Autodesk Inventor part; units mm, degrees
ref_plane "Work Plane2" through (0, 0, 6.858) normal (0, 0, 1) x (1, 0, 0)
ref_plane "YZ Plane" through (0, 0, 0) normal (1, 0, 0) x (0, 1, 0)
ref_plane "XZ Plane" through (0, 0, 0) normal (0, 1, 0) x (-1, 0, 0)
sketch "Sketch1" plane through (0, 0, 0) normal (0, 0, 1) x (1, 0, 0)
  circle A0 centre (0, 0) radius 2.159
  dimension "d0" = 4.318
extrude "Extrusion1" add sketch "Sketch1" along normal blind 15.748
sketch "Sketch2" plane through (0, 0, 15.748) normal (0, 0, 1) x (1, 0, 0)
  circle A0 centre (0, 0) radius 1.275
  dimension "d23" = 2.55
extrude "Extrusion2" cut sketch "Sketch2" against normal blind 15.24
sketch "Sketch6" plane through (0, 0, 15.748) normal (0, 0, 1) x (1, 0, 0)
  line L0 (-1.6256, 0.5334) -> (1.6256, 0.5334)
  line L1 (1.6256, 0.5334) -> (1.6256, -0.5334)
  line L2 (1.6256, -0.5334) -> (-1.6256, -0.5334)
  line L3 (-1.6256, -0.5334) -> (-1.6256, 0.5334)
  point P0 (0, 0)
  dimension "d24" = 0.5334
  dimension "d25" = 0.5334
  dimension "d26" = 1.6256
  dimension "d27" = 1.6256
extrude "Extrusion6" cut sketch "Sketch6" against normal blind 8.89
ref_plane "Work Plane2" through (0, 0, 6.858) normal (0, 0, 1) x (1, 0, 0)
sketch "Sketch7" plane through (0, 0, 6.858) normal (0, 0, 1) x (1, 0, 0)
  line L0 (1.6428, -0.5334) -> (1.1581, -0.5334)
  line L1 (-1.6428, 0.5334) -> (-0.5334, 0.5334)
  arc A0 (1.6428, -0.5334) -> (-0.5334, 1.6428) centre (0, 0) ccw
  arc A1 (-1.6428, 0.5334) -> (0.5334, -1.6428) centre (0, 0) ccw
  line L2 (1.6256, -0.5334) -> (0.5334, -0.5334)
  line L3 (0.5334, -0.5334) -> (0.5334, -1.6428)
  line L4 (-0.5334, 0.5334) -> (-0.5334, 1.6428)
extrude "Extrusion7" cut sketch "Sketch7" along normal blind 5.588
sketch "Sketch8" plane through (0, 0, 0) normal (0, 0, -1) x (-1, 0, 0)
  line L0 (-3.8846, 4.0845) -> (4.056, 4.0845)
  line L1 (4.056, 4.0845) -> (4.056, 0)
  line L2 (4.056, 0) -> (-3.8846, 0)
  line L3 (-3.8846, 0) -> (-3.8846, 4.0845)
  point P0 (0, 0)
extrude "Extrusion8" cut sketch "Sketch8" against normal blind 25.4
properties part number "Snap-Twist Idea F"
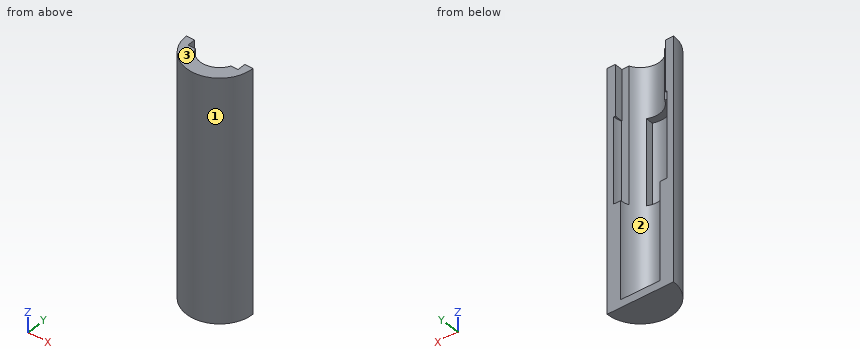
Input: part model. Units: mm. Frame: model coordinates. Face numbers are marked on the shaded views. Round coordinates to 2 decimals unless told otherwise and drop trailing zeros. Loops run counter-clockwise (first coordinate to the right, second up) from the corner with the lowest first, then second, coordinate; pieces in that order, holes last. Notation, with made-up numbers: (6, -7.5) -> (43, -7.5) arc R31 ccw to (43, 21.5) -> close; hole circle Ø9 at (-6.5, 72). An arc over 180 degrees is marked (long way). One line per item, written item: value.
(1) Section C-C (z = 5.5). Return the cut outline in (x, y) (3 decimals).
Geometry check:
outline: (-2.159, 0) arc R2.159 ccw to (2.159, 0) -> (1.275, 0) arc R1.275 cw to (-1.275, 0) -> close
(2) Pin query (flat end, axial travel): pin 1 (2 mm diameter, centred on x = 1.5, z = 2.5, fed in from -Y); pin 2 (0.6 mm diameter, centred on x = 0, y = -0.5, fed in from +Z). Return the tip coordinate at first contact, or that it passes through.
Geometry check:
pin 1: y = -2.1
pin 2: z = 0.51
(3) Material intervals for line 1 (X direction, y = -0.05, z = 13.25); line 2 (X direction, y = -1.2, z = 10.25); line 3 (Z direction, x = 1.05, y = -0.65), sorted ascending. Write a range as [from, to].
Geometry check:
line 1: [-2.16, -1.63], [1.63, 2.16]
line 2: [-1.79, -1.24], [0.53, 1.79]
line 3: [0, 0.51]
(4) Section B-B (z = 11.5). Return the cut outline in (x, y) (3 decimals).
Geometry check:
outline: (-2.159, 0) arc R2.159 ccw to (2.159, 0) -> (1.727, 0) arc R1.727 cw to (1.643, -0.533) -> (1.158, -0.533) arc R1.275 cw to (0.533, -1.158) -> (0.533, -1.643) arc R1.727 cw to (-1.727, 0) -> close
(5) Section A-A (x = 0). Return the cut outline in (y, z) (3 decimals), plus the area to 3 significant figures.
Geometry check:
outline: (-2.159, 0) -> (0, 0) -> (0, 0.508) -> (-1.275, 0.508) -> (-1.275, 6.858) -> (-1.727, 6.858) -> (-1.727, 12.446) -> (-1.275, 12.446) -> (-1.275, 15.748) -> (-2.159, 15.748) -> close
area: 12.0 mm2
(6) Mould query, pull axis X, two halves, no side actions, for the marked faces 1, 2 and 3. Classes: pulls with the +X half, pulls with the -X half, needs draft (parallel to the pull), parting line crosses it, or undercut.
Geometry check:
face 1: parting line crosses it
face 2: undercut
face 3: needs draft
